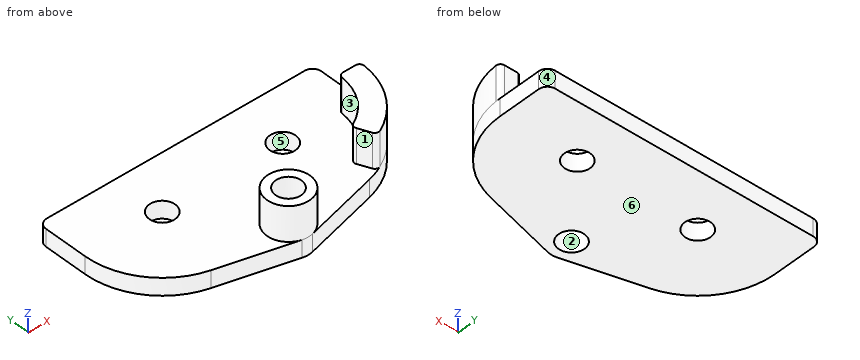
from build123d import *

# Parameters (mm, degrees)
SKETCH_2_R      = 1.5
EXTRUDE_1_DEPTH = 2
EXTRUDE_2_DEPTH = 4
FILLET_1_R      = 1
FILLET_4_R      = 0.5
SKETCH_4_R      = 2.5
SKETCH_4_R_2    = 1.5
EXTRUDE_3_DEPTH = 4


with BuildPart() as part:
    # 草图2 → 凸台-拉伸1 (new body)
    with BuildSketch(Plane.XY):
        with BuildLine():
            Line((7, 6), (-7, 6))
            Line((-7, 6), (-16, 6))
            Line((-16, 6), (-16, 0))
            ThreePointArc((-16, 0), (-14.108952351, -5.519311231), (-9.230489674, -8.71922679))
            Line((-9.230489674, -8.71922679), (-0.619580465, -10.922007442))
            ThreePointArc((-0.619580465, -10.922007442), (0, -11), (0.619580465, -10.922007442))
            Line((0.619580465, -10.922007442), (9.230489674, -8.71922679))
            ThreePointArc((9.230489674, -8.71922679), (14.108952351, -5.519311231), (16, 0))
            Line((16, 0), (16, 6))
            Line((16, 6), (7, 6))
        make_face()
        with Locations((0, -8.5)):
            Circle(SKETCH_2_R, mode=Mode.SUBTRACT)
        with Locations((7, 0)):
            Circle(SKETCH_2_R, mode=Mode.SUBTRACT)
        with Locations(Location((-7, 0, 0), (0, 0, 180))):
            Circle(SKETCH_2_R, mode=Mode.SUBTRACT)
    extrude(amount=EXTRUDE_1_DEPTH)

    # 草图3 → 凸台-拉伸2 (add)
    with BuildSketch(Plane.XY.offset(2)):
        with BuildLine():
            Line((13.5, 0), (16, 0))
            ThreePointArc((16, 0), (14.527522767, -4.933193793), (10.591910889, -8.252161909))
            Line((10.591910889, -8.252161909), (9.594157864, -5.959894712))
            ThreePointArc((9.594157864, -5.959894712), (12.43654422, -3.562862184), (13.5, 0))
        make_face()
    extrude(amount=EXTRUDE_2_DEPTH)

    # 圆角1
    fillet_1_edges = [part.edges().sort_by_distance(p)[0] for p in [
        (-16, 6, 1),
        (16, 6, 1),
    ]]
    fillet(fillet_1_edges, radius=FILLET_1_R)

    # 圆角4
    fillet_4_edges = [part.edges().sort_by_distance(p)[0] for p in [
        (10.591910889, -8.252161909, 4),
        (16, 0, 4),
        (13.5, 0, 4),
        (9.594157864, -5.959894712, 4),
    ]]
    fillet(fillet_4_edges, radius=FILLET_4_R)

    # 草图4 → 凸台-拉伸3 (add)
    with BuildSketch(Plane.XY.offset(2)):
        with Locations(Location((0, -8.5, 0), (0, 0, 255.650730884))):
            Circle(SKETCH_4_R)
        with Locations((0, -8.5)):
            Circle(SKETCH_4_R_2, mode=Mode.SUBTRACT)
    extrude(amount=EXTRUDE_3_DEPTH)


solid = part.part
Check sheet for the modelled part. Datum: model origin and axes. Units: mm. Face numbers are marked on the shaded views. A direction names the side the tool comes from. Round coordinates to 2 decimals unless told otherwise and drop trailing zeros. Loops run counter-clockwise (first coordinate to the right, second up) from the corner with the lowest first, then second, coordinate; pieces in that order, holes last. Notation, with made-up numbers: M -40,45 L 2,45 A30 cw 2,78 Z; hole C -21.75,-13.5 d10. An arc over 180 degrees is marked long. One line per item, written item: value.
(1) Release check for a two-part mould opening along X. For the marked faces 4, 5 and 6 record: +X half, -X half, draft (parallel to the pull), parting line (faces both ways), or undercut.
Computed values:
face 4: +X half
face 5: undercut
face 6: draft
(2) Sectioned sample at D-D, the plane y = -9.25. Record the cut outline in (x, z).
Computed values:
outline: M -7.16,0 L -1.3,0 L -1.3,6 L -2.38,6 L -2.38,2 L -7.16,2 Z; M 1.3,0 L 7.16,0 L 7.16,2 L 2.38,2 L 2.38,6 L 1.3,6 Z
(3) Sectioned sample at B-B, the plane z = 1. Record the cut outline in (x, y), then the cut area to 3 significant figures.
Computed values:
outline: M -16,0 A9 ccw -9.23,-8.72 L -0.62,-10.92 A2.5 ccw 0.62,-10.92 L 9.23,-8.72 A9 ccw 16,0 L 16,5 A1 ccw 15,6 L -15,6 A1 ccw -16,5 Z; hole C -7,0 d3; hole C 0,-8.5 d3; hole C 7,0 d3
area: 441 mm^2
(4) Sectioned sample at A-A, the plane z = 2.75. Record the cut outline in (x, y).
Computed values:
outline: C 0,-8.5 d5; M 9.79,-6.4 L 10.39,-7.78 A0.5 ccw 11.07,-8.03 A9 ccw 15.98,-0.53 A0.5 ccw 15.49,0 L 13.98,0 A0.5 ccw 13.48,-0.46 A6.5 cw 10.01,-5.76 A0.5 ccw Z; hole C 0,-8.5 d3
(5) Depth check by flat-ended pin: pin 1 Ø3 at (x, z) = (10, 1.5) entering from -Y; pin 2 Ø3 at (y, z) = (-7.5, 4.5) entering from +X; pin 3 Ø2 at (y, z) = (-3, 2) entering from -X. Enter the tip coordinate at first touch or a pass-through.
Computed values:
pin 1: stops at y = -8.91
pin 2: stops at x = 13.71
pin 3: stops at x = -15.77
(6) Sectioned sample at C-C, the plane x = 6.5. Record the cut outline in (y, z), then the cut area to 3 significant figures.
Computed values:
outline: M -9.42,0 L -1.41,0 L -1.41,2 L -9.42,2 Z; M 1.41,0 L 6,0 L 6,2 L 1.41,2 Z
area: 25.2 mm^2
(7) Access from +Z, -Z, +X, -X, +Y, -Y to the whole of each face (thin tool, end or side, straight path). Record for the marked faces 1, 2 and 3.
Computed values:
face 1: +Z, -Y
face 2: +Z, -Z
face 3: +Z, -X, +Y
(8) Thickness scan on line 1 (Y direction, x = 0, z = 2.6); line 2 (X direction, y = -1, z = 0.75); line 3 (Z direction, x = -8.5, y = -3). Record the ranges inside material, lowest first.
Computed values:
line 1: y = -11 to -10, -7 to -6
line 2: x = -15.94 to -8.12, -5.88 to 5.88, 8.12 to 15.94
line 3: z = 0 to 2
